from build123d import *

# Parameters (mm, degrees)
F1_DEPTH       = 6.35
F2_R           = 3.81
F3_DEPTH       = 6.35
F5_D           = 1.9304
F5_CSINK_D     = 4.2672
F5_CSINK_ANGLE = 82
F7_D           = 2.032


with BuildPart() as f1:
    # F0 (on Top) → F1 (new body)
    with BuildSketch(Plane.XY):
        with BuildLine():
            Line((-6.35, 34.29), (-6.35, 12.7))
            ThreePointArc((-6.35, 12.7), (-4.4901280605, 17.1901280605), (0, 19.05))
            Line((0, 19.05), (0, 27.94))
            ThreePointArc((0, 27.94), (-4.4901280605, 29.7998719395), (-6.35, 34.29))
        make_face()
        with BuildLine():
            ThreePointArc((0, 19.05), (4.4901280605, 17.1901280605), (6.35, 12.7))
            Line((6.35, 12.7), (6.35, 32.3486101727))
            Line((6.35, 32.3486101727), (5.2643885857, 30.739125063))
            ThreePointArc((5.2643885857, 30.739125063), (2.9811444237, 28.6832827853), (0, 27.94))
            Line((0, 27.94), (0, 19.05))
        make_face()
        with BuildLine():
            ThreePointArc((-5.2643885857, 37.840874937), (-6.0725352004, 36.146560325), (-6.35, 34.29))
            ThreePointArc((-6.35, 34.29), (-4.4901280605, 29.7998719395), (0, 27.94))
            Line((0, 27.94), (0, 34.29))
            Line((0, 34.29), (3.550874937, 39.5543885857))
            ThreePointArc((3.550874937, 39.5543885857), (-1.2116371206, 40.5233326149), (-5.2643885857, 37.840874937))
        make_face()
        with BuildLine():
            Line((5.2643885857, 30.739125063), (6.35, 32.3486101727))
            Line((6.35, 32.3486101727), (6.35, 34.29))
            ThreePointArc((6.35, 34.29), (5.6067172147, 37.2711444237), (3.550874937, 39.5543885857))
            Line((3.550874937, 39.5543885857), (0, 34.29))
            Line((0, 34.29), (0, 27.94))
            ThreePointArc((0, 27.94), (2.9811444237, 28.6832827853), (5.2643885857, 30.739125063))
        make_face()
        with BuildLine():
            Line((6.35, 34.29), (6.35, 32.3486101727))
            Line((6.35, 32.3486101727), (27.9899881828, 64.4312120116))
            ThreePointArc((27.9899881828, 64.4312120116), (26.2764745341, 73.2464755344), (17.4612110113, 71.5329618857))
            Line((17.4612110113, 71.5329618857), (-5.2643885857, 37.840874937))
            ThreePointArc((-5.2643885857, 37.840874937), (-1.2116371206, 40.5233326149), (3.550874937, 39.5543885857))
            ThreePointArc((3.550874937, 39.5543885857), (5.6067172147, 37.2711444237), (6.35, 34.29))
        make_face()
        with BuildLine():
            Line((0, 12.7), (0, 6.35))
            ThreePointArc((0, 6.35), (4.4901280605, 8.2098719395), (6.35, 12.7))
            ThreePointArc((6.35, 12.7), (4.4901280605, 17.1901280605), (0, 19.05))
            Line((0, 19.05), (0, 12.7))
        make_face()
        with BuildLine():
            ThreePointArc((-6.35, 12.7), (-4.4901280605, 8.2098719395), (0, 6.35))
            Line((0, 6.35), (0, 12.7))
            Line((0, 12.7), (0, 19.05))
            ThreePointArc((0, 19.05), (-4.4901280605, 17.1901280605), (-6.35, 12.7))
        make_face()
        with BuildLine():
            ThreePointArc((6.35, 12.7), (4.4901280605, 8.2098719395), (0, 6.35))
            ThreePointArc((0, 6.35), (-4.4901280605, 8.2098719395), (-6.35, 12.7))
            Line((-6.35, 12.7), (-6.35, 0))
            ThreePointArc((-6.35, 0), (0, -6.35), (6.35, 0))
            Line((6.35, 0), (6.35, 12.7))
        make_face()
    extrude(amount=F1_DEPTH)

    # F2 (on face) → F3 (join)
    with BuildSketch(Plane.XY.offset(6.35)):
        with Locations((0, 12.7)):
            Circle(F2_R)
    extrude(amount=F3_DEPTH)

    # F5 (through all)
    with Locations(Plane.XY.offset(12.7)):
        with Locations((0, 12.7)):
            CounterSinkHole(F5_D / 2, F5_CSINK_D / 2, counter_sink_angle=F5_CSINK_ANGLE)

    # F7 (through all)
    with Locations(Plane.XY.offset(6.35)):
        with Locations((0, 0)):
            Hole(F7_D / 2)


solid = f1.part
Model file for the job. Use its own axes, mm. A direction names the side the tool comes from. Give positions to 0.01 mm unless a question says otherwise; leave off trailing zeros. Loops run counter-clockwise (first coordinate to the right, second up) from the corner with the lowest first, then second, coordinate; pieces in that order, holes last.
1) Saw through at D-D (z = 8.25). Write the cut outline in (x, y), plus the area to 3 significant figures.
2) Wall check: line 1 (Y direction, x = 0, z = 6.5); line 2 (Y direction, x = 0, z = 3.25); line 3 (Y direction, x = 0.5, z = 1.25). Give the ranges that are in metal, low to high.
3) Saw through at B-B (z = 1.75). Write the cut outline in (x, y), plus the area to 3 significant figures.
4) Tool access for faces 1 (the cylindrical face through (26.39, 73.17, 3.13)), 2 (the cylindrical face through (-0.83, 8.98, 9.48)), 3 (the flat face through (6.35, 16, 3)): list every direction of +Z, -Z, +X, -X, +Y, -Y with a clear straight run to the whole face (end or side of a thin tool).
5) Pull direction X, two halves, no side cores. Call faces 4 (the flat face through (7, 35, 6.35)), 5 (the cylindrical face through (0.126, 13.657, 5.598)), 6 (the flat face through (17.02, 48.17, 3.13)): +X half, -X half, draft (parallel to the pull), parting line (faces both ways), or undercut.
6) Saw through at C-C (x = 0). Write the cut outline in (y, z), plus the area to 3 significant figures.
7) Flat gauge pins, fed straight in: pin 1 Ø3 at (x, z) = (10.5, 4) entering from +Y; pin 2 Ø1.2 at (x, y) = (0, 12.7) entering from +Z; pin 3 Ø8 at (x, y) = (20.5, 49) entering from +Z; pin 4 Ø3 at (y, z) = (15.5, 4) entering from +X. Where does each tip first touch, or does it go through?
8) Saw through at A-A (y = 12.7). Write the cut outline in (x, z).
Answer block:
1. outline: circle Ø7.62 at (0, 12.7); hole circle Ø1.93 at (0, 12.7)
1. area: 42.7 mm2
2. line 1: y = 8.89 to 11.73, 13.67 to 16.51
2. line 2: y = -6.35 to -1.02, 1.02 to 11.73, 13.67 to 45.65
2. line 3: y = -6.33 to -0.88, 0.88 to 11.87, 13.53 to 46.39
3. outline: (-6.35, 0) arc R6.35 ccw to (6.35, 0) - (6.35, 32.35) - (27.99, 64.43) arc R6.35 ccw to (17.46, 71.53) - (-5.26, 37.84) arc R6.35 ccw to (-6.35, 34.29) - close; hole circle Ø2.03 at (0, 0); hole circle Ø1.93 at (0, 12.7)
3. area: 1,070 mm2
4. face 1: +Z, -Z
4. face 2: +Z
4. face 3: +Z, -Z, +X, -Y
5. face 4: draft
5. face 5: undercut
5. face 6: +X half
6. outline: (-6.35, 0) - (-1.02, 0) - (-1.02, 6.35) - (-6.35, 6.35) - close; (1.02, 0) - (11.73, 0) - (11.73, 11.36) - (10.57, 12.7) - (8.89, 12.7) - (8.89, 6.35) - (1.02, 6.35) - close; (13.67, 0) - (45.65, 0) - (45.65, 6.35) - (16.51, 6.35) - (16.51, 12.7) - (14.83, 12.7) - (13.67, 11.36) - close
6. area: 340 mm2
7. pin 1: stops at y = 63.44
7. pin 2: passes through
7. pin 3: stops at z = 6.35
7. pin 4: stops at x = 6.35
8. outline: (-6.35, 0) - (-0.97, 0) - (-0.97, 11.36) - (-2.13, 12.7) - (-3.81, 12.7) - (-3.81, 6.35) - (-6.35, 6.35) - close; (0.97, 0) - (6.35, 0) - (6.35, 6.35) - (3.81, 6.35) - (3.81, 12.7) - (2.13, 12.7) - (0.97, 11.36) - close
